from build123d import *

# Parameters (mm, degrees)
SKETCH_W        = 175
SKETCH_H        = 65
PAD_DEPTH       = 5
SKETCH001_R     = 20
PAD001_DEPTH    = 4
SKETCH002_R     = 9.5
POCKET_DEPTH    = 9.01
PAD002_DEPTH    = 65
PAD003_DEPTH    = 5
PAD004_DEPTH    = 5
SKETCH006_R     = 4.15
POCKET001_DEPTH = 2
POCKET001_TAPER = 45
SKETCH007_R     = 2.1
POCKET002_DEPTH = 5


with BuildPart() as part:
    # Sketch → Pad (new body)
    with BuildSketch(Plane.XY):
        Rectangle(SKETCH_W, SKETCH_H)
    extrude(amount=PAD_DEPTH)

    # Sketch001 (on Face6 of Pad) → Pad001 (join)
    with BuildSketch(Plane.XY.offset(5)):
        with Locations((57.5, 0)):
            Circle(SKETCH001_R)
    extrude(amount=PAD001_DEPTH)

    # Sketch002 (on Face8 of Pad001) → Pocket (cut)
    with BuildSketch(Plane.XY.offset(9)):
        with Locations((57.5, 0)):
            Circle(SKETCH002_R)
    extrude(amount=-POCKET_DEPTH, mode=Mode.SUBTRACT)

    # Sketch003 (on Face6 of Pocket) → Pad002 (join)
    with BuildSketch(Plane.XZ.offset(32.5)):
        Polygon((-88.5, 5), (-87.5, -60), (-82.5, -60), (-82.5, 5), align=None)
    extrude(amount=-PAD002_DEPTH)

    # Sketch004 (on Face3 of Pad002) → Pad003 (join)
    with BuildSketch(Plane(origin=(0, 32.5, 0), x_dir=(-1, 0, 0), z_dir=(0, 1, 0))):
        Polygon((-87.5, 5), (-87.5, 0), (82.5, -60), (87.5, -60), (88.5, 5), align=None)
    extrude(amount=-PAD003_DEPTH)

    # Sketch005 (on Face23 of Pad003) → Pad004 (join)
    with BuildSketch(Plane.XZ.offset(32.5)):
        Polygon((-88.5, 5), (-87.5, -60), (-82.5, -60), (87.5, 0), (87.5, 5), align=None)
    extrude(amount=-PAD004_DEPTH)

    # Sketch006 (on Face21 of Pad004) → Pocket001 (cut)
    with BuildSketch(Plane.YZ.offset(-82.5)):
        with Locations((0, -25)):
            Circle(SKETCH006_R)
        with Locations((-12.5, -50)):
            Circle(SKETCH006_R)
        with Locations((12.5, -50)):
            Circle(SKETCH006_R)
    extrude(amount=-POCKET001_DEPTH, taper=POCKET001_TAPER, mode=Mode.SUBTRACT)

    # Sketch007 (on Face41 of Pocket001) → Pocket002 (cut)
    with BuildSketch(Plane.YZ.offset(-84.5)):
        with Locations((0, -25)):
            Circle(SKETCH007_R)
        with Locations((12.5, -50)):
            Circle(SKETCH007_R)
        with Locations((-12.5, -50)):
            Circle(SKETCH007_R)
    extrude(amount=-POCKET002_DEPTH, mode=Mode.SUBTRACT)


solid = part.part
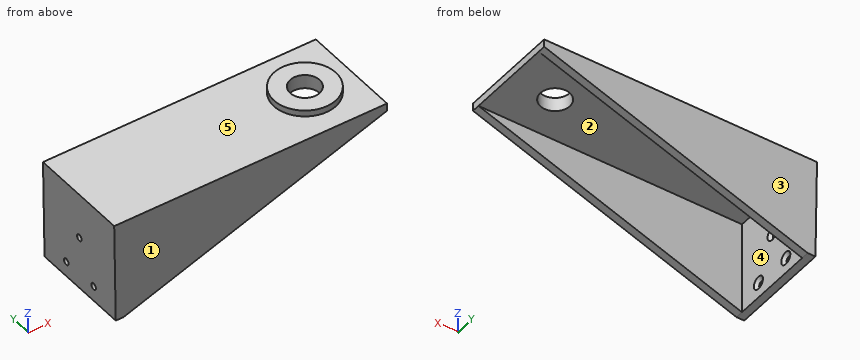
Here's how the part is built. I have some questions about the finished solid (model axes, mm). Face numbers are marked on the shaded views. A direction names the side the tool comes from. Coordinates: 2 decimals unless noted, no trailing zeros. Loops run counter-clockwise (first coordinate to the right, second up) from the corner with the lowest first, then second, coordinate; pieces in that order, holes last. Notation, with made-up numbers: (11.5, 6.25) -> (53.5, 6.25) arc R11 cw to (53.5, 14.25) -> close; hole circle Ø6 at (6, 67). An arc over 180 degrees is marked (long way). Use one line per item in the form item = value. Start each with the question number.
(1) If we section it at C-C (z = -3): Please give me the cut outline in (x, y), then the cut area to 3 significant figures.
(2) If we section it at B-B (y = 0): Please give me the cut outline in (x, z), then the cut area to 3 significant figures.
(3) If we section it at D-D (y = 12.5): Please give me the cut outline in (x, z).
(4) Will these pins go through, and if not, where does the flat tip stop? pin 1 (6 mm diameter, centred on x = 35.5, y = -5, fed in from -Z); pin 2 (4.5 mm diameter, centred on y = -1, z = -26, fed in from +X); pin 3 (2.5 mm diameter, centred on y = 12.5, z = -50, fed in from +X) (3 decimals); pin 4 (5 mm diameter, centred on y = 0, z = -25, fed in from -X).
(5) On a 3-axis mill with a long thin cutter (end or side, diameter ignored), from which of +Z, -Z, +X, -X, +Y, -Y can I reach the whole of each face in a straight line? I mean the marked faces 1 and 2. Say none if no direction works.
(6) Please list where these lines run through material, in increasing order: line 1 along Y through (x, z) = (-86, -50); line 2 along Z through (x, y) = (-87, 0); line 3 along Y through (x, z) = (-86, -25).
(7) If we section it at A-A (x = 57.5): Please give me the cut outline in (y, z).
(8) We'd pull the mould along Y, two halves only. Please class the marked faces 3, 4 and 5: pulls with the +Y half, pulls with the -Y half, needs draft (parallel to the pull), parting line crosses it, or undercut.
Verdict:
q1.outline = (-88.38, -32.5) -> (79, -32.5) -> (79, -27.5) -> (-82.5, -27.5) -> (-82.5, 27.5) -> (79, 27.5) -> (79, 32.5) -> (-88.38, 32.5) -> close
q1.area = 2,000 mm²
q2.outline = (-88.5, 5) -> (-88.07, -22.9) -> (-84.5, -22.9) -> (-84.5, -22.85) -> (-82.5, -20.85) -> (-82.5, 0) -> (48, 0) -> (48, 9) -> (37.5, 9) -> (37.5, 5) -> close; (-88.01, -27.1) -> (-87.5, -60) -> (-82.5, -60) -> (-82.5, -29.15) -> (-84.5, -27.15) -> (-84.5, -27.1) -> close; (67, 0) -> (87.5, 0) -> (87.5, 5) -> (77.5, 5) -> (77.5, 9) -> (67, 9) -> close
q2.area = 1,170 mm²
q3.outline = (-88.5, 5) -> (-87.69, -47.9) -> (-84.5, -47.9) -> (-84.5, -47.85) -> (-82.5, -45.85) -> (-82.5, 0) -> (87.5, 0) -> (87.5, 5) -> (73.11, 5) -> (73.11, 9) -> (41.89, 9) -> (41.89, 5) -> close; (-87.62, -52.1) -> (-87.5, -60) -> (-82.5, -60) -> (-82.5, -54.15) -> (-84.5, -52.15) -> (-84.5, -52.1) -> close
q4.pin_1 = 0
q4.pin_2 = -82.99
q4.pin_3 = through
q4.pin_4 = -88.08
q5.face_1 = +Z, -Z, +X, -X, -Y
q5.face_2 = -Z, +X
q6.line_1 = -32.5 to -14.6, -10.4 to 10.4, 14.6 to 32.5
q6.line_2 = -60 to -27.1, -22.9 to 5
q6.line_3 = -32.5 to -2.1, 2.1 to 32.5
q7.outline = (-32.5, -10.59) -> (-27.5, -10.59) -> (-27.5, 0) -> (-9.5, 0) -> (-9.5, 9) -> (-20, 9) -> (-20, 5) -> (-32.5, 5) -> close; (9.5, 0) -> (27.5, 0) -> (27.5, -10.59) -> (32.5, -10.59) -> (32.5, 5) -> (20, 5) -> (20, 9) -> (9.5, 9) -> close
q8.face_3 = pulls with the +Y half
q8.face_4 = undercut
q8.face_5 = needs draft
